For this review, take the finished solid that the model builds, in its own axes (mm). Give positions to 0.01 mm unless a question says otherwise; leave off trailing zeros. Loops run counter-clockwise (first coordinate to the right, second up) from the corner with the lowest first, then second, coordinate; pieces in that order, holes last.
```python
from build123d import *

# Parameters (mm, degrees)
F1_DEPTH = 7
F2_D     = 8.5
F3_SIZE  = 1


with BuildPart() as f1:
    # F0 (on Front) → F1 (new body)
    with BuildSketch(Plane.XZ):
        Polygon((3.4641016151, 6), (-3.4641016151, 6), (-6.9282032303, 0), (-3.4641016151, -6), (3.4641016151, -6), (6.9282032303, 0), align=None)
    extrude(amount=F1_DEPTH)

    # F2 (through all)
    with Locations(Plane(origin=(0, 0, 0), x_dir=(1, 0, 0), z_dir=(0, 1, 0))):
        with Locations((0, 0)):
            Hole(F2_D / 2)

    # F3
    f3_edges = [f1.edges().sort_by_distance(p)[0] for p in [
        (0, -7, 6),
        (-5.196152, -7, 3),
        (-5.196152, -7, -3),
        (0, -7, -6),
        (5.196152, -7, -3),
        (5.196152, -7, 3),
        (5.196152, 0, 3),
        (0, 0, 6),
        (-5.196152, 0, 3),
        (-5.196152, 0, -3),
        (0, 0, -6),
        (5.196152, 0, -3),
    ]]
    chamfer(f3_edges, length=F3_SIZE)


solid = f1.part
```
Q1. For pin 1 Ø1 at (y, z) = (-5.5, -3) entering from +X, flat-tipped, find the tip position at first contact; note if it passes through.
Answers:
pin 1: stops at x = 5.48
Q2. For probe 1 along Z at (x, y) = (0, -4.75); probe 2 along Z at (x, y) = (3.75, -5.5); probe 3 along X at (y, z) = (-2.75, -1), list the stretches that pass through material, from the lowest coordinate up.
Answers:
probe 1: z = -6 to -4.25, 4.25 to 6
probe 2: z = -5.5 to -2, 2 to 5.5
probe 3: x = -6.35 to -4.13, 4.13 to 6.35
Q3. Consider section D-D on z = 4.75. Give the boundary of the cut face in (x, y).
Answers:
outline: (-4.19, -6) - (-3.03, -7) - (3.03, -7) - (4.19, -6) - (4.19, -1) - (3.03, 0) - (-3.03, 0) - (-4.19, -1) - close
Q4. Consider section A-A on x = 0. Give the boundary of the cut face in (y, z), plus the area to 3 significant figures.
Answers:
outline: (-7, -5) - (-6, -6) - (-1, -6) - (0, -5) - (0, -4.25) - (-7, -4.25) - close; (-7, 4.25) - (0, 4.25) - (0, 5) - (-1, 6) - (-6, 6) - (-7, 5) - close
area: 22.5 mm2
Q5. Consider section B-B on y = -2.5. Give the boundary of the cut face in (x, z).
Answers:
outline: (-6.93, 0) - (-3.46, -6) - (3.46, -6) - (6.93, 0) - (3.46, 6) - (-3.46, 6) - close; hole circle Ø8.5 at (0, 0)
Q6. Consider section C-C on z = 0.5. Give the boundary of the cut face in (x, y), plus the area to 3 significant figures.
Answers:
outline: (-6.64, -6) - (-5.48, -7) - (-4.22, -7) - (-4.22, 0) - (-5.48, 0) - (-6.64, -1) - close; (4.22, -7) - (5.48, -7) - (6.64, -6) - (6.64, -1) - (5.48, 0) - (4.22, 0) - close
area: 31.6 mm2
